Build history of the part. All positions in model axes, mm. Face numbers are marked on the shaded views. A direction names the side the tool comes from. Coordinates: 2 decimals unless noted, no trailing zeros. Loops run counter-clockwise (first coordinate to the right, second up) from the corner with the lowest first, then second, coordinate; pieces in that order, holes last.
Item 1: Cut at B-B (y = 18). List the corners of the cut face in (x, z), and give its area (3 significant figures).
Item 2: Cut at C-C (z = 29). List the corners of the cut face in (x, y).
Item 3: Drill centre lines: line 1 along X through (y, z) = (39, -22); line 2 along Y through (x, z) = (-63.9, 20); line 3 along X through (y, z) = (11, -5). Where is each one in solid material? Low to high.
Item 4: Cut at D-D (x = 34). List the corners of the cut face in (y, z), and give its area (3 significant figures).
Item 5: Cut at A-A (z = -30). List the corners of the cut face in (x, y), and give its area (3 significant figures).
Item 6: 3-axis set-ups, long thin cutter, end or side, ignore diameter. For the marked faces 4 and 5: which of +Z, -Z, +X, -X, +Y, -Y reach the whole face in a straight line?
Item 7: Flat gauge pins, fed straight in: pin 1 (5 mm diameter, centred on x = 20, y = 30.5, fed in from +Z); pin 2 (8 mm diameter, centred on x = 55.5, y = 19.5, fed in from +Z); pin 3 (10 mm diameter, centred on x = 6, z = 10.5, fed in from +Y). Where does each tip first touch, or does it go through?
Item 8: Mould opens along Z. For the marked faces 1, 2 and 3 say: released by +Z, released by -Z, zero draft, split by the parting line, or undercut.
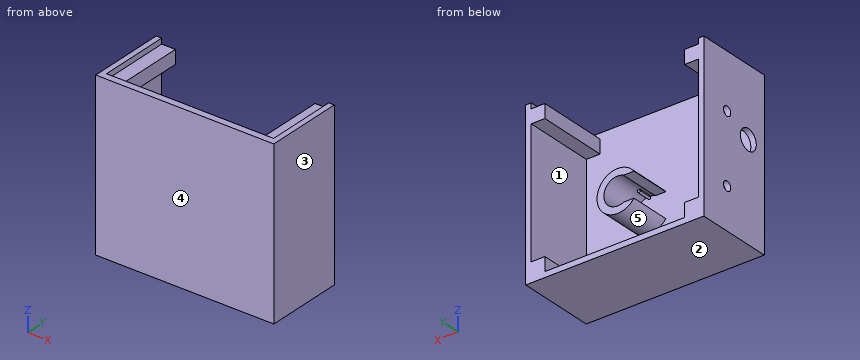
from build123d import *

# Parameters (mm, degrees)
SKETCH4_W           = 130
SKETCH4_H           = 120
BOSS_EXTRUDE1_DEPTH = 5
BOSS_EXTRUDE2_DEPTH = 52
SKETCH6_W           = 10
SKETCH6_H           = 10
BOSS_EXTRUDE3_DEPTH = 52
SKETCH7_R           = 7.5
CUT_EXTRUDE1_DEPTH  = 5
SKETCH8_R           = 15
SKETCH8_R_2         = 10
BOSS_EXTRUDE4_DEPTH = 30
BOSS_EXTRUDE5_DEPTH = 10
SKETCH10_W          = 15
SKETCH10_H          = 18
CUT_EXTRUDE2_DEPTH  = 30
SKETCH11_R          = 3.41
CUT_EXTRUDE3_DEPTH  = 5


with BuildPart() as part:
    # Sketch4 → Boss-Extrude1 (new body)
    with BuildSketch(Plane(origin=(0, 0, 0), x_dir=(1, 0, 0), z_dir=(0, 1, 0))):
        Rectangle(SKETCH4_W, SKETCH4_H)
    extrude(amount=BOSS_EXTRUDE1_DEPTH)

    # Sketch5 → Boss-Extrude2 (add)
    with BuildSketch(Plane(origin=(0, 5, 0), x_dir=(1, 0, 0), z_dir=(0, 1, 0))):
        Polygon((-65, -60), (-65, 60), (65, 60), (65, -60), (61, -60), (61, 56), (-61, 56), (-61, -60), align=None)
    extrude(amount=BOSS_EXTRUDE2_DEPTH)

    # Sketch6 → Boss-Extrude3 (add)
    with BuildSketch(Plane(origin=(0, 5, 0), x_dir=(1, 0, 0), z_dir=(0, 1, 0))):
        with Locations((-56, 51)):
            Rectangle(SKETCH6_W, SKETCH6_H)
        with Locations((56, 51)):
            Rectangle(SKETCH6_W, SKETCH6_H)
        with Locations((56, -51)):
            Rectangle(SKETCH6_W, SKETCH6_H)
        with Locations((-56, -51)):
            Rectangle(SKETCH6_W, SKETCH6_H)
    extrude(amount=BOSS_EXTRUDE3_DEPTH)

    # Sketch7 → Cut-Extrude1 (cut)
    with BuildSketch(Plane.ZY.offset(65)):
        with Locations((10, 15)):
            Circle(SKETCH7_R)
    extrude(amount=-CUT_EXTRUDE1_DEPTH, mode=Mode.SUBTRACT)

    # Sketch8 → Boss-Extrude4 (add)
    with BuildSketch(Plane(origin=(0, 5, 0), x_dir=(1, 0, 0), z_dir=(0, 1, 0))):
        with Locations(Location((15, 5, 0), (0, 0, 90))):
            Circle(SKETCH8_R)
        with Locations(Location((15, 5, 0), (0, 0, 270))):
            Circle(SKETCH8_R_2, mode=Mode.SUBTRACT)
    extrude(amount=BOSS_EXTRUDE4_DEPTH)

    # Sketch9 → Boss-Extrude5 (add)
    with BuildSketch(Plane(origin=(0, 5, 0), x_dir=(1, 0, 0), z_dir=(0, 1, 0))):
        with BuildLine():
            Line((14, -4), (14, -5.590084182))
            Line((14, -5.590084182), (16, -5.590084182))
            Line((16, -5.590084182), (16, -4))
            ThreePointArc((16, -4), (15, -3), (14, -4))
        make_face()
        with BuildLine():
            Line((14, 14), (14, 15.761522781))
            Line((14, 15.761522781), (16, 15.761522781))
            Line((16, 15.761522781), (16, 14))
            ThreePointArc((16, 14), (15, 13), (14, 14))
        make_face()
    extrude(amount=BOSS_EXTRUDE5_DEPTH)

    # Sketch10 → Cut-Extrude2 (cut)
    with BuildSketch(Plane(origin=(0, 35, 0), x_dir=(1, 0, 0), z_dir=(0, 1, 0))):
        with Locations((5.5, 5)):
            Rectangle(SKETCH10_W, SKETCH10_H)
    extrude(amount=-CUT_EXTRUDE2_DEPTH, mode=Mode.SUBTRACT)

    # Sketch11 → Cut-Extrude3 (cut)
    with BuildSketch(Plane.ZY.offset(65)):
        with Locations((-30, 35)):
            Circle(SKETCH11_R)
        with Locations((20, 35)):
            Circle(SKETCH11_R)
    extrude(amount=-CUT_EXTRUDE3_DEPTH, mode=Mode.SUBTRACT)


solid = part.part
Filled sheet:
1. outline: (-65, -60) - (65, -60) - (65, 60) - (61, 60) - (61, 56) - (51, 56) - (51, 46) - (61, 46) - (61, -46) - (51, -46) - (51, -56) - (-51, -56) - (-51, -46) - (-61, -46) - (-61, 3.13) - (-65, 3.13) - close; (-65, 16.87) - (-61, 16.87) - (-61, 46) - (-51, 46) - (-51, 56) - (-61, 56) - (-61, 60) - (-65, 60) - close; (3, -14) arc R15 ccw (long way) to (3, 4) - (10.64, 4) arc R10 cw (long way) to (10.64, -14) - close
1. area: 2,080 mm2
2. outline: (-65, 0) - (65, 0) - (65, 57) - (61, 57) - (61, 5) - (-61, 5) - (-61, 57) - (-65, 57) - close
3. line 1: x = -65 to -61, 61 to 65
3. line 2: y = 0 to 31.59, 38.41 to 57
3. line 3: x = -65 to -61, 25 to 30, 61 to 65
4. outline: (0, -60) - (57, -60) - (57, -56) - (5, -56) - (5, 60) - (0, 60) - close
4. area: 808 mm2
5. outline: (-65, 0) - (65, 0) - (65, 57) - (61, 57) - (61, 5) - (-61, 5) - (-61, 31.59) - (-65, 31.59) - close; (-65, 38.41) - (-61, 38.41) - (-61, 57) - (-65, 57) - close
5. area: 1,040 mm2
6. face 4: +Z, -Z, +X, -X, -Y
6. face 5: +Y
7. pin 1: stops at z = 9.79
7. pin 2: stops at z = 56
7. pin 3: stops at y = 35
8. face 1: undercut
8. face 2: released by -Z
8. face 3: zero draft
